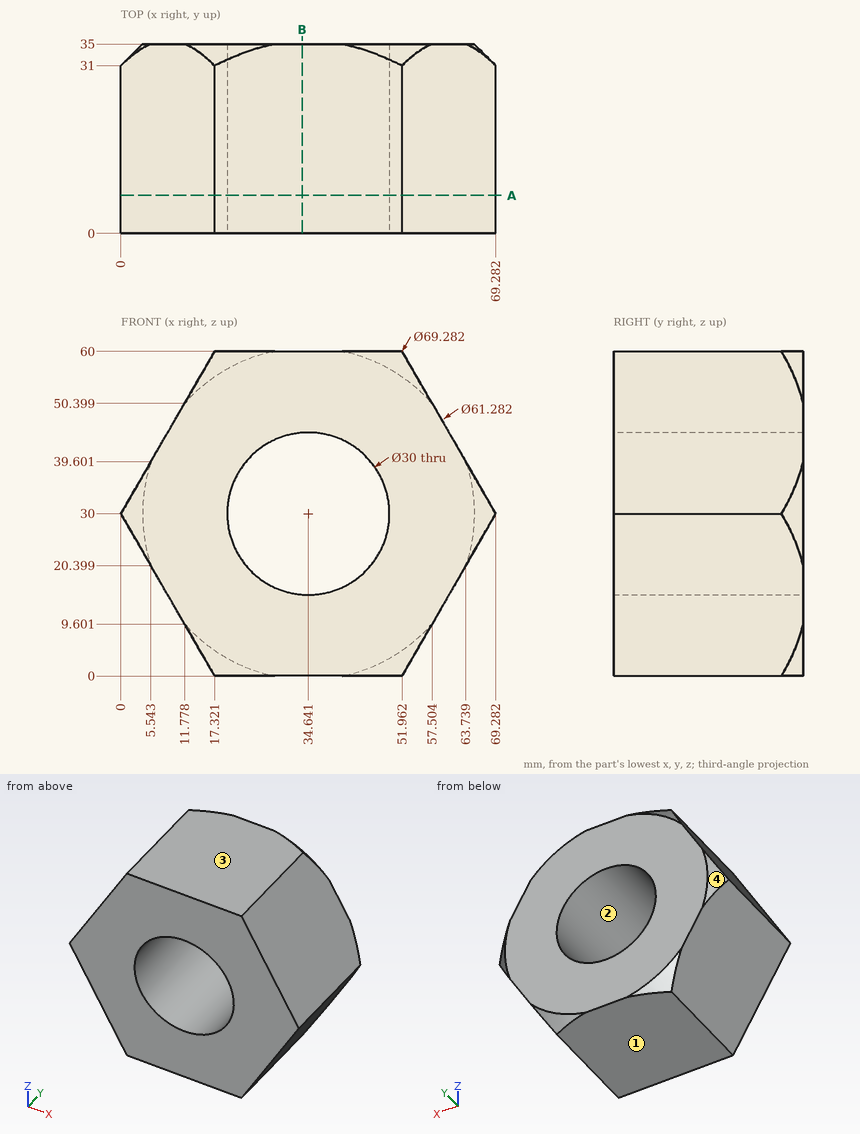
Can you work these out from the drawing? Everything is in mm from the part's minimum corner. Coordinates: 2 decimals unless noted, no trailing zeros. Write each loop counter-clockwise with the first axis right and the second up, starting at its lowest first coordinate (ties: lowest second). Pieces come first, ordered by that corner, then holes. Notation, with made-up numbers: (83.5, 37) - (136.5, 37) arc R21 ccw to (136.5, 64) - close; hole circle Ø8 at (-5, -34). An arc over 180 degrees is marked (long way). One line per item, written item: value.
1) We'd pull the mould along Z, two halves only. Please class the marked faces 1, 2, 3 and 4: pulls with the +Z half, pulls with the -Z half, needs draft (parallel to the pull), parting line crosses it, or undercut.
Model answer:
face 1: pulls with the -Z half
face 2: undercut
face 3: pulls with the +Z half
face 4: parting line crosses it
2) Suppose I cut it at A-A on y = 7. Write out the boundary of the cut face in (x, z), and give its area (3 significant figures).
Model answer:
outline: (0, 30) - (17.32, 0) - (51.96, 0) - (69.28, 30) - (51.96, 60) - (17.32, 60) - close; hole circle Ø30 at (34.64, 30)
area: 2,410 mm²
3) I'm going to push flat-ended pins straight in: P1, Ø1, axis at y = 15.5, z = 43, coming from the -X side; P2, Ø6, axis at y = 16, z = 10.5, coming from the +X side (1 decimal); P3, Ø3, axis at y = 18.5, z = 26, coming from the -X side. Where does each tip first touch, or does it pass through?
Model answer:
P1: stops at x = 7.22
P2: stops at x = 59.8
P3: stops at x = 1.44
4) Suppose I cut it at B-B on x = 33.5. Write out the boundary of the cut face in (y, z).
Model answer:
outline: (0, 0) - (35, 0) - (35, 15.04) - (0, 15.04) - close; (0, 44.96) - (35, 44.96) - (35, 60) - (0, 60) - close
5) I need wall thicknesses on line 1 along X through (y, z) = (19, 34) (1 decimal); line 2 along X through (y, z) = (9.5, 43) (1 decimal); line 3 along Z through (x, y) = (43.5, 17) (1 decimal). Which ranges of each line are inside material? Lowest first, please.
Model answer:
line 1: x = 2.3 to 20.2, 49.1 to 67
line 2: x = 7.5 to 27.2, 42.1 to 61.8
line 3: z = 0 to 17.9, 42.1 to 60
